Verification items for this drawing (mm, ordinates from the low corner). Round coordinates to 2 decimals unless told otherwise and drop trailing zeros. Order: outer loops, then holes, each group sorted by start corner. A loop starts at its lowest first (then second) coordinate and runs counter-clockwise, first axis right, second up. Notation, with made-up numbers: (61, -11) -> (92, -11) arc R16 cw to (92, 12) -> close; hole circle Ø11 at (-15.75, -7.5). An arc over 180 degrees is marked (long way). Use a Markdown table: item, result. Add a question column.
Item 1: Sectioned sample at C-C, the plane x = 7.25. Record the cut outline in (y, z), and give its area (3 significant figures).
Item 2: Material ranges on probe 1 along X at (y, z) = (0.55, 11); probe 2 along Y at (x, z) = (8, 33.5); probe 3 along Z at (x, y) = (15.25, 2.15), recorded low to high. Write a range as [from, to].
Item 3: Sectioned sample at B-B, the plane z = 20. Record the cut outline in (x, y).
Item 4: Sectioned sample at D-D, the plane z = 37. Record the cut outline in (x, y), and give its area (3 significant figures).
Item 5: Mould release check, pull along X, two halves, no side actions. Record for the marked faces 1, 2, 3 and 4: pulls with the +X half, pulls with the -X half, needs draft (parallel to the pull), parting line crosses it, or undercut.
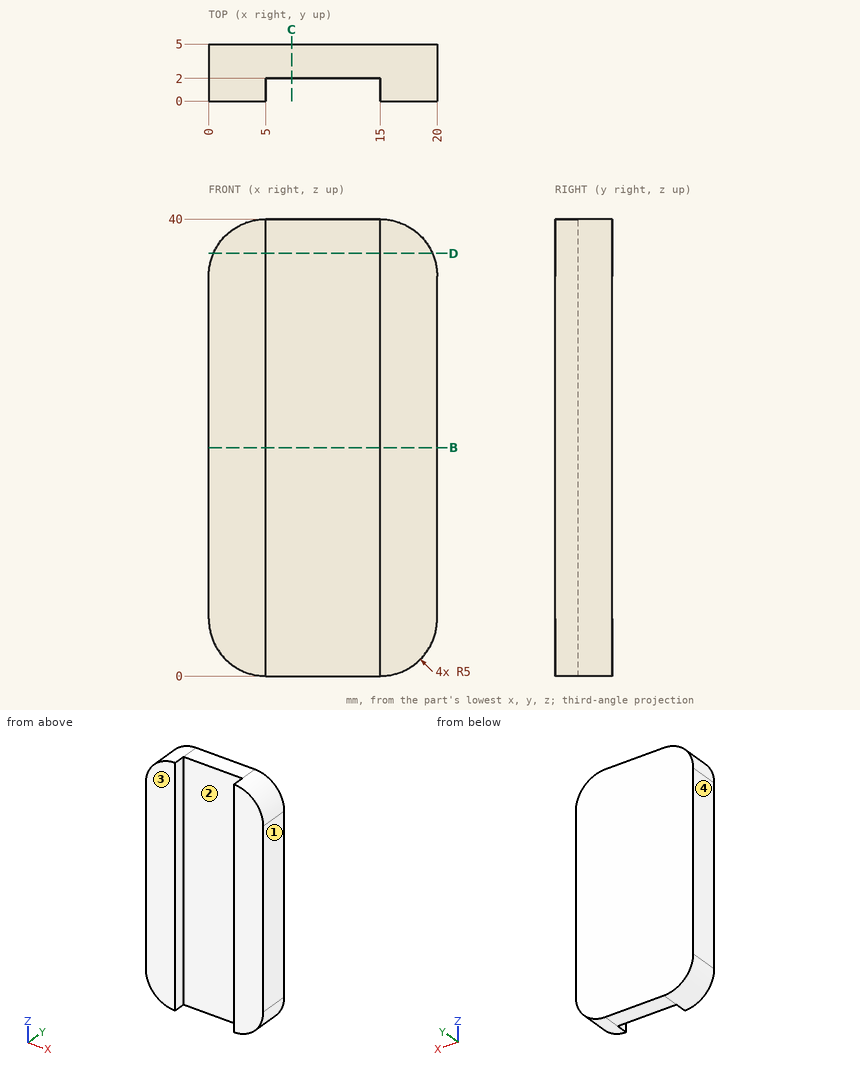
Found:
| question | item | result |
|---|---|---|
| 1 | outline | (2, 0) -> (5, 0) -> (5, 40) -> (2, 40) -> close |
| 1 | area | 120 mm2 |
| 2 | probe 1 | x = [0, 5], [15, 20] |
| 2 | probe 2 | y = [2, 5] |
| 2 | probe 3 | z = [0.01, 39.99] |
| 3 | outline | (0, 0) -> (5, 0) -> (5, 2) -> (15, 2) -> (15, 0) -> (20, 0) -> (20, 5) -> (0, 5) -> close |
| 4 | outline | (0.42, 0) -> (5, 0) -> (5, 2) -> (15, 2) -> (15, 0) -> (19.58, 0) -> (19.58, 5) -> (0.42, 5) -> close |
| 4 | area | 75.8 mm2 |
| 5 | face 1 | pulls with the +X half |
| 5 | face 2 | undercut |
| 5 | face 3 | needs draft |
| 5 | face 4 | pulls with the -X half |
